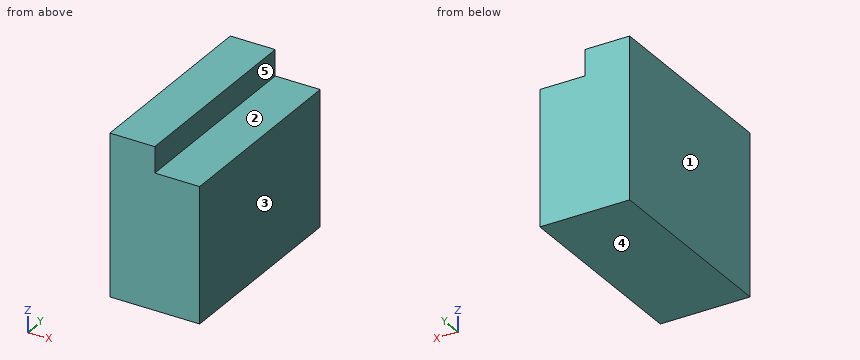
from build123d import *

# Parameters (mm, degrees)
F0_W     = 1447.8
F0_H     = 1181.1
F1_DEPTH = 330.2
F2_W     = 1447.8
F2_H     = 990.6
F3_DEPTH = 330.2


with BuildPart() as f1:
    # F0 (on Right) → F1 (new body)
    with BuildSketch(Plane.YZ):
        Rectangle(F0_W, F0_H)
    extrude(amount=F1_DEPTH)

    # F2 (on face) → F3 (join)
    with BuildSketch(Plane.YZ.offset(330.2)):
        with Locations((0, -95.25)):
            Rectangle(F2_W, F2_H)
    extrude(amount=F3_DEPTH)


solid = f1.part
Could you check a few things on this model? Use its own coordinates, in mm. Face numbers are marked on the shaded views. A direction names the side the tool comes from. Give positions to 0.01 mm unless a question says otherwise; leave off trailing zeros. Write each loop counter-clockwise with the first axis right and the second up, starting at its lowest first coordinate (ties: lowest second). Pieces come first, ordered by that corner, then holes. Notation, with made-up numbers: (79.25, 62.5) - (83.25, 62.5) arc R22 ccw to (83.25, 100.5) - close; hole circle Ø10 at (26.25, 4.5). An arc over 180 degrees is marked (long way). Use CSV: the item, a comma, the result in double quotes. Start each with the question number.
Item 1: I want a section at A-A, the plane y = -122.5. Please give me the cut outline in (x, z).
Item 2: I want a section at B-B, the plane x = 619.5. Please give me the cut outline in (y, z), then the cut area to 3 significant figures.
Item 3: I want a section at C-C, the plane z = 471.5. Please give me the cut outline in (x, y).
Item 4: If I drill on line 1 along X through (y, z) = (-145, 475); line 2 along Z through (x, y) = (494, 599), over which ranges is the centre line in solid material (lowest first)?
Item 5: For the marked faces 4 and 5, which set-ups out of +Z, -Z, +X, -X, +Y, -Y let a thin tool reach every point of the face, with its end or its side?
Item 6: If we mould it in two halves opening along X, with no side actions, what happens to the marked faces 1, 2 and 3? For each: pulls with the +X half, pulls with the -X half, needs draft (parallel to the pull), parting line crosses it, or undercut.
Findings:
1,outline,"(0, -590.55) - (660.4, -590.55) - (660.4, 400.05) - (330.2, 400.05) - (330.2, 590.55) - (0, 590.55) - close"
2,outline,"(-723.9, -590.55) - (723.9, -590.55) - (723.9, 400.05) - (-723.9, 400.05) - close"
2,area,"1,430,000 mm2"
3,outline,"(0, -723.9) - (330.2, -723.9) - (330.2, 723.9) - (0, 723.9) - close"
4,line 1,"x = 0 to 330.2"
4,line 2,"z = -590.55 to 400.05"
5,face 4,"-Z, +X, -X, +Y, -Y"
5,face 5,"+Z, +X, +Y, -Y"
6,face 1,"pulls with the -X half"
6,face 2,"needs draft"
6,face 3,"pulls with the +X half"
